```python
from build123d import *

# Parameters (mm, degrees)
SKETCH1_R           = 2
BOSS_EXTRUDE1_DEPTH = 5


with BuildPart() as part:
    # Sketch1 → Boss-Extrude1 (new body)
    with BuildSketch(Plane.XY):
        with BuildLine():
            ThreePointArc((-25.85, -9.9), (-27.617766953, -9.167766953), (-28.35, -7.4))
            Line((-28.35, -7.4), (-28.35, 9.9))
            Line((-28.35, 9.9), (-20.15, 9.9))
            Line((-20.15, 9.9), (-20.15, -9.9))
            Line((-20.15, -9.9), (-25.85, -9.9))
        make_face()
        with Locations((-24.25, -5)):
            Circle(SKETCH1_R, mode=Mode.SUBTRACT)
        with Locations((-24.25, 5)):
            Circle(SKETCH1_R, mode=Mode.SUBTRACT)
        with BuildLine():
            Line((-28.35, 9.9), (-20.15, 9.9))
            Line((-20.15, 9.9), (20.15, 9.9))
            Line((20.15, 9.9), (28.35, 9.9))
            Line((28.35, 9.9), (28.35, 17.4))
            ThreePointArc((28.35, 17.4), (27.617766953, 19.167766953), (25.85, 19.9))
            Line((25.85, 19.9), (-25.85, 19.9))
            ThreePointArc((-25.85, 19.9), (-27.617766953, 19.167766953), (-28.35, 17.4))
            Line((-28.35, 17.4), (-28.35, 9.9))
        make_face()
        with BuildLine():
            ThreePointArc((28.35, -7.4), (27.617766953, -9.167766953), (25.85, -9.9))
            Line((25.85, -9.9), (20.15, -9.9))
            Line((20.15, -9.9), (20.15, 9.9))
            Line((20.15, 9.9), (28.35, 9.9))
            Line((28.35, 9.9), (28.35, -7.4))
        make_face()
        with Locations((24.25, 5)):
            Circle(SKETCH1_R, mode=Mode.SUBTRACT)
        with Locations((24.25, -5)):
            Circle(SKETCH1_R, mode=Mode.SUBTRACT)
    extrude(amount=BOSS_EXTRUDE1_DEPTH)


solid = part.part
```
Could you check a few things on this model? Use its own coordinates, in mm. A direction names the side the tool comes from. Round coordinates to 2 decimals unless told otherwise and drop trailing zeros. Write each loop counter-clockwise with the first axis right and the second up, starting at its lowest first coordinate (ties: lowest second). Pieces come first, ordered by that corner, then holes. Notation, with made-up numbers: M 81.25,-10.75 L 122.25,-10.75 A20 ccw 122.25,27.25 Z; hole C 12.5,-3.75 d2. An arc over 180 degrees is marked long. Answer in a Markdown table with one row per item. Add a question column.
Q1. Imagine slicing it at A-A (y = 5). Please give me the cut outline in (x, z), then the cut area to 3 significant figures.
Q2. Imagine slicing it at D-D (x = 16). Please give me the cut outline in (y, z), then the cut area to 3 significant figures.
Q3. If we mould it in two halves opening along Y, with no side actions, what happens to faces 3 (the flat face through (0, 12, 0)), 4 (the flat face through (0, 9.9, 2)), 5 (the cylindrical face through (22.663, -6.217, 2.465)), 6 (the cylindrical face through (-25.837, -6.217, 2.465))? For each: +Y half, -Y half, draft (parallel to the pull), parting line (faces both ways), or undercut.
Q4. On a 3-axis mill with a long thin cutter (end or side, diameter ignored), from which of +Z, -Z, +X, -X, +Y, -Y can I reach the whole of each face in a straight line? I mean faces 1 (the flat face through (-20.15, 0, 2)), 2 (the cylindrical face through (22.252, 5.088, 2.465)). Say none if no direction works.
Q5. Imagine slicing it at C-C (z = 2.9). Please give me the cut outline in (x, y).
Q6. If I drill on line 1 (Y direction, x = 24.25, z = 3.1); line 2 (X direction, y = -7.25, z = 1.4); line 3 (X direction, y = -5.75, z = 2.2), over which ranges is the centre line in solid material (lowest first)? Write a range as from..to.
Q7. Imagine slicing it at B-B (x = 24.25). Please give me the cut outline in (y, z).
Q8. Will these pins go through, and if not, where does the flat tip stop? pin 1 Ø10 at (x, y) = (-15, 4) entering from -Z; pin 2 Ø2.5 at (x, z) = (5, 1.5) entering from -Y.
Values:
| question | item | result |
|---|---|---|
| 1 | outline | M -28.35,0 L -26.25,0 L -26.25,5 L -28.35,5 Z; M -22.25,0 L -20.15,0 L -20.15,5 L -22.25,5 Z; M 20.15,0 L 22.25,0 L 22.25,5 L 20.15,5 Z; M 26.25,0 L 28.35,0 L 28.35,5 L 26.25,5 Z |
| 1 | area | 42.0 mm^2 |
| 2 | outline | M 9.9,0 L 19.9,0 L 19.9,5 L 9.9,5 Z |
| 2 | area | 50.0 mm^2 |
| 3 | face 3 | draft |
| 3 | face 4 | -Y half |
| 3 | face 5 | undercut |
| 3 | face 6 | undercut |
| 4 | face 1 | +Z, -Z, -Y |
| 4 | face 2 | +Z, -Z |
| 5 | outline | M -28.35,-7.4 A2.5 ccw -25.85,-9.9 L -20.15,-9.9 L -20.15,9.9 L 20.15,9.9 L 20.15,-9.9 L 25.85,-9.9 A2.5 ccw 28.35,-7.4 L 28.35,17.4 A2.5 ccw 25.85,19.9 L -25.85,19.9 A2.5 ccw -28.35,17.4 Z; hole C -24.25,-5 d4; hole C -24.25,5 d4; hole C 24.25,-5 d4; hole C 24.25,5 d4 |
| 6 | line 1 | -9.9..-7, -3..3, 7..19.9 |
| 6 | line 2 | -28.35..-20.15, 20.15..28.35 |
| 6 | line 3 | -28.35..-26.1, -22.4..-20.15, 20.15..22.4, 26.1..28.35 |
| 7 | outline | M -9.9,0 L -7,0 L -7,5 L -9.9,5 Z; M -3,0 L 3,0 L 3,5 L -3,5 Z; M 7,0 L 19.9,0 L 19.9,5 L 7,5 Z |
| 8 | pin 1 | through |
| 8 | pin 2 | y = 9.9 |
